Input: dimensioned drawing with shaded views. Units: mm. Origin: part minimum x, y, z. Coordinates: 2 decimals unless noted, no trailing zeros. Write each loop counter-clockwise with the first axis right and the second up, starting at its lowest first coordinate (ties: lowest second). Pieces come first, ordered by that corner, then holes. Notation, with made-up numbers: (83, 22) -> (131, 22) arc R24 cw to (131, 33) -> close; hole circle Ø9 at (-19, 74.5). An arc over 180 degrees is marked (long way). One line per item, written item: value. Start each with the question number.
1. Section query A-A, the plane z = 2. Output: boundary loops of the cut face in (x, y), and give its area (3 significant figures).
2. Section query C-C, the plane y = 2.25. Output: boundary loops of the cut face in (x, z).
3. Section query D-D, the plane y = 7.5. Output: boundary loops of the cut face in (x, z).
4. Mould query, pull axis X, two halves, no side actions, for the marked faces 1, 2, 3 and 4. Classes: released by +X, released by -X, zero draft, split by the parting line, or undercut.
5. Section query B-B, the plane x = 12.5. Output: boundary loops of the cut face in (y, z).
6. First-contact query: P1, Ø1.8, axis at x = 3, z = 2, coming from the -Y side; P2, Ø1, axis at x = 13, z = 3.5, coming from the +Y side; P3, Ø1.6, axis at x = 17, z = 2, coming from the +Y side. Flat tips, straight axial feed; report the tip coordinate or a pass-through.
7. Line query: line 1 (Z direction, x = 17, y = 1.8); line 2 (Y direction, x = 10, z = 2.8); line 3 (Y direction, x = 11.5, z = 3.05). Output: solid intervals per line, ascending.
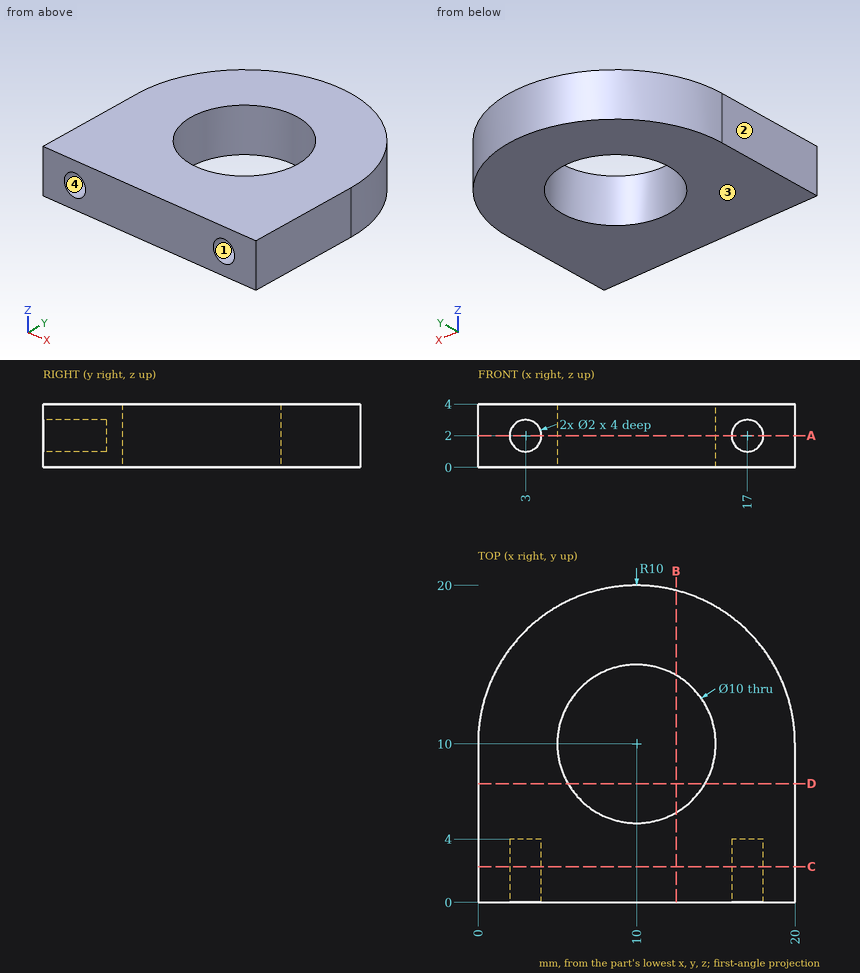
Computed values:
1. outline: (0, 0) -> (2, 0) -> (2, 4) -> (4, 4) -> (4, 0) -> (16, 0) -> (16, 4) -> (18, 4) -> (18, 0) -> (20, 0) -> (20, 10) arc R10 ccw to (0, 10) -> close; hole circle Ø10 at (10, 10)
1. area: 263 mm²
2. outline: (0, 0) -> (20, 0) -> (20, 4) -> (0, 4) -> close; hole circle Ø2 at (3, 2); hole circle Ø2 at (17, 2)
3. outline: (0, 0) -> (5.67, 0) -> (5.67, 4) -> (0, 4) -> close; (14.33, 0) -> (20, 0) -> (20, 4) -> (14.33, 4) -> close
4. face 1: undercut
4. face 2: released by -X
4. face 3: zero draft
4. face 4: undercut
5. outline: (0, 0) -> (5.67, 0) -> (5.67, 4) -> (0, 4) -> close; (14.33, 0) -> (19.68, 0) -> (19.68, 4) -> (14.33, 4) -> close
6. P1: stops at y = 4
6. P2: stops at y = 19.68
6. P3: stops at y = 17.85
7. line 1: z = 0 to 1, 3 to 4
7. line 2: y = 0 to 5, 15 to 20
7. line 3: y = 0 to 5.23, 14.77 to 19.89
